```python
from build123d import *

# Parameters (mm, degrees)
SKETCH1_R           = 1.5
SKETCH1_R_2         = 1.44463942
SKETCH1_R_3         = 1.75
SKETCH1_W           = 23.332723566
SKETCH1_H           = 13.458477976
SKETCH1_W_2         = 20.606585233
SKETCH1_H_2         = 10.826007204
BOSS_EXTRUDE1_DEPTH = 3


with BuildPart() as part:
    # Sketch1 → Boss-Extrude1 (new body)
    with BuildSketch(Plane(origin=(0, 0, 0), x_dir=(1, 0, 0), z_dir=(0, 1, 0))):
        Polygon((-72.5, -35), (72.5, -35), (72.5, 35), (-2.5, 35), (-2.5, 115), (-72.5, 115), (-72.5, 35), align=None)
        with Locations(Location((3.654827994, -29.242640687, 0), (0, 0, 270))):
            Circle(SKETCH1_R, mode=Mode.SUBTRACT)
        with Locations(Location((12.140109368, -20.757359313, 0), (0, 0, 270))):
            Circle(SKETCH1_R_2, mode=Mode.SUBTRACT)
        with Locations(Location((53.338095075, -29.242640687, 0), (0, 0, 270))):
            Circle(SKETCH1_R, mode=Mode.SUBTRACT)
        with Locations(Location((61.823376449, -20.757359313, 0), (0, 0, 270))):
            Circle(SKETCH1_R, mode=Mode.SUBTRACT)
        with Locations(Location((-16.814355015, 100.757359313, 0), (0, 0, 270))):
            Circle(SKETCH1_R, mode=Mode.SUBTRACT)
        with Locations(Location((-8.329073641, 109.242640687, 0), (0, 0, 270))):
            Circle(SKETCH1_R, mode=Mode.SUBTRACT)
        with Locations(Location((-13.69982199, 1.5, 0), (0, 0, 270))):
            Circle(SKETCH1_R, mode=Mode.SUBTRACT)
        with Locations(Location((59.109237961, 1.5, 0), (0, 0, 270))):
            Circle(SKETCH1_R, mode=Mode.SUBTRACT)
        with Locations(Location((-63.584566194, -27.710636817, 0), (0, 0, 270))):
            Circle(SKETCH1_R_3, mode=Mode.SUBTRACT)
        with Locations(Location((-43.584566194, -27.710636817, 0), (0, 0, 270))):
            Circle(SKETCH1_R_3, mode=Mode.SUBTRACT)
        with Locations(Location((-43.584566194, 32.289363183, 0), (0, 0, 270))):
            Circle(SKETCH1_R_3, mode=Mode.SUBTRACT)
        with Locations(Location((-63.584566194, 32.289363183, 0), (0, 0, 270))):
            Circle(SKETCH1_R_3, mode=Mode.SUBTRACT)
        with Locations(Location((-68.740395312, 53.009730632, 0), (0, 0, 270))):
            Circle(SKETCH1_R, mode=Mode.SUBTRACT)
        with Locations(Location((-68.740395312, 93.009730632, 0), (0, 0, 270))):
            Circle(SKETCH1_R, mode=Mode.SUBTRACT)
        with Locations(Location((-8.740395312, 93.009730632, 0), (0, 0, 270))):
            Circle(SKETCH1_R, mode=Mode.SUBTRACT)
        with Locations(Location((-8.740395312, 53.009730632, 0), (0, 0, 270))):
            Circle(SKETCH1_R, mode=Mode.SUBTRACT)
        with Locations((-20.406757095, 22.7)):
            Rectangle(SKETCH1_W, SKETCH1_H, mode=Mode.SUBTRACT)
        with Locations((53.46751152, 21.383764614)):
            Rectangle(SKETCH1_W_2, SKETCH1_H_2, mode=Mode.SUBTRACT)
    extrude(amount=BOSS_EXTRUDE1_DEPTH)


solid = part.part
```
Geometry check sheet. Reference: the model listing, model coordinates, mm. Coordinates: 2 decimals unless noted, no trailing zeros. Order: outer loops, then holes, each group sorted by start corner. A loop starts at its lowest first (then second) coordinate and runs counter-clockwise, first axis right, second up. Notation, with made-up numbers: M 21.5,-14.75 L 67.5,-14.75 A18 ccw 67.5,4.25 Z; hole C 64,80.25 d11. An arc over 180 degrees is marked long. Answer as a JSON object with one key per item and string values.
Q1. Scan lines: line 1 (X direction, y = 0.8, z = -26.5); line 2 (X direction, y = 0.85, z = -29); line 3 (Z direction, x = -63.5, y = 1.2). Record each from-to range of solid material in increasing order.
Results are:
{"line 1": "x = -72.5 to -32.07, -8.74 to 43.16, 63.77 to 72.5", "line 2": "x = -72.5 to -32.07, -8.74 to 72.5", "line 3": "z = -115 to -34.04, -30.54 to 25.96, 29.46 to 35"}
Q2. Cross-section at D-D on x = 24. Record the cut outline in (y, z), and give its area (3 significant figures).
Results are:
{"outline": "M 0,-35 L 3,-35 L 3,35 L 0,35 Z", "area": "210 mm²"}
Q3. Cross-section at C-C on z = -80. Record the cut outline in (x, y), and give its area (3 significant figures).
Results are:
{"outline": "M -72.5,0 L -2.5,0 L -2.5,3 L -72.5,3 Z", "area": "210 mm²"}
Q4. Depth check by flat-ended pin: pin 1 Ø1 at (x, y) = (27.5, 0.5) entering from -Z. Enter the tip coordinate at first touch or a pass-through.
Results are:
{"pin 1": "stops at z = -35"}
Q5. Cross-section at B-B on y = 2. Give the number of separate pieces and of enclosed holes in the cut face, and give its area (3 significant figures).
Results are:
{"separate pieces": "1", "enclosed holes": "18", "area": "15,100 mm²"}
Q6. Cross-section at A-A on x = -22. Record the cut outline in (y, z).
Results are:
{"outline": "M 0,-115 L 3,-115 L 3,-29.43 L 0,-29.43 Z; M 0,-15.97 L 3,-15.97 L 3,35 L 0,35 Z"}
